```python
from build123d import *

# Parameters (mm, degrees)
CROQUIS1_W              = 75
CROQUIS1_H              = 160
CROQUIS1_R              = 3
SALIENTE_EXTRUIR1_DEPTH = 3
REDONDEO1_R             = 6


with BuildPart() as part:
    # Croquis1 → Saliente-Extruir1 (new body)
    with BuildSketch(Plane.XY):
        Rectangle(CROQUIS1_W, CROQUIS1_H)
        with Locations((-29.5, 72)):
            Circle(CROQUIS1_R, mode=Mode.SUBTRACT)
        with Locations((29.5, 72)):
            Circle(CROQUIS1_R, mode=Mode.SUBTRACT)
        with Locations((-29.5, -72)):
            Circle(CROQUIS1_R, mode=Mode.SUBTRACT)
        with Locations((29.5, -72)):
            Circle(CROQUIS1_R, mode=Mode.SUBTRACT)
    extrude(amount=SALIENTE_EXTRUIR1_DEPTH)

    # Redondeo1
    redondeo1_edges = [part.edges().sort_by_distance(p)[0] for p in [
        (-37.5, 80, 1.5),
        (37.5, 80, 1.5),
        (37.5, -80, 1.5),
        (-37.5, -80, 1.5),
    ]]
    fillet(redondeo1_edges, radius=REDONDEO1_R)


solid = part.part
```
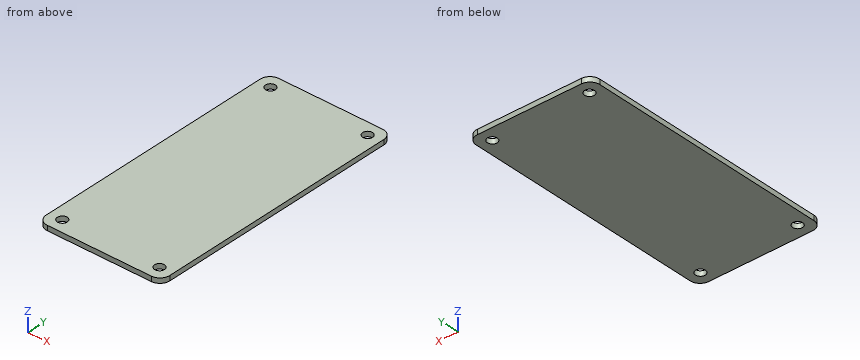
The model under review builds one solid part; all positions refer to its coordinate system, in mm. Give positions to 0.01 mm unless a question says otherwise; leave off trailing zeros. Loops run counter-clockwise (first coordinate to the right, second up) from the corner with the lowest first, then second, coordinate; pieces in that order, holes last. Notation, with made-up numbers: (57.25, -31.5) - (85.25, -31.5) arc R17 cw to (85.25, 0.5) - close; hole circle Ø9 at (-33.5, 88.5). An arc over 180 degrees is marked (long way). Answer as a JSON object with one key per item and string values.
Q1. Add section B-B on x = 29.5. State the section outline as (y, z) points.
Worked out:
{"outline": "(-80, 0) - (-75, 0) - (-75, 3) - (-80, 3) - close; (-69, 0) - (69, 0) - (69, 3) - (-69, 3) - close; (75, 0) - (80, 0) - (80, 3) - (75, 3) - close"}
Q2. To check wall thickness, follow line 1 along Y through (x, z) = (29.5, 1.15); line 2 along Y through (x, z) = (28, 0.1); line 3 along Y through (x, z) = (33.5, 1.25). State the ranges of each line that lie inside material, in increasing order.
Worked out:
{"line 1": "y = -80 to -75, -69 to 69, 75 to 80", "line 2": "y = -80 to -74.6, -69.4 to 69.4, 74.6 to 80", "line 3": "y = -79.66 to 79.66"}
Q3. Insertion check: pin 1 (2 mm diameter, centred on x = -12.5, y = -19.5, fed in from -Z); pin 2 (5 mm diameter, centred on x = -29.5, y = 72, fed in from +Z). Each pin has a flat end and moves straight along its axis. Give the tip position at first contact, or say it passes through.
Worked out:
{"pin 1": "stops at z = 0", "pin 2": "passes through"}
Q4. Add section A-A on y = -72. State the section outline as (x, z) points.
Worked out:
{"outline": "(-37.5, 0) - (-32.5, 0) - (-32.5, 3) - (-37.5, 3) - close; (-26.5, 0) - (26.5, 0) - (26.5, 3) - (-26.5, 3) - close; (32.5, 0) - (37.5, 0) - (37.5, 3) - (32.5, 3) - close"}
